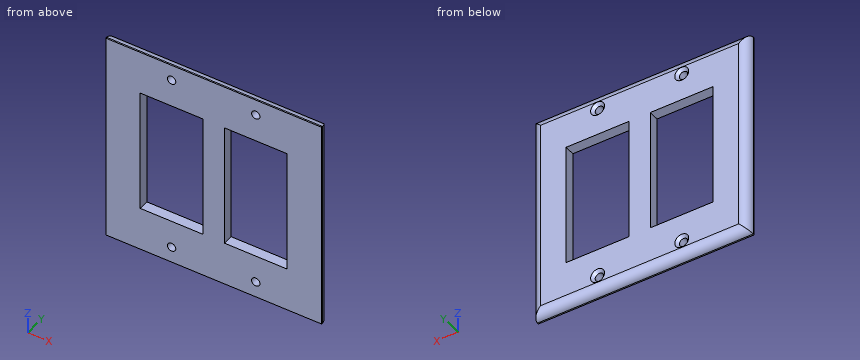
from build123d import *

# Parameters (mm, degrees)
SKETCH1_W           = 116
SKETCH1_H           = 114.3
SKETCH1_R           = 2.25
SKETCH1_W_2         = 33.75
SKETCH1_H_2         = 67
BOSS_EXTRUDE1_DEPTH = 5.5
FILLET1_R           = 4.75
CHAMFER1_SIZE       = 1.5


with BuildPart() as part:
    # Sketch1 → Boss-Extrude1 (new body)
    with BuildSketch(Plane(origin=(0, 0, 0), x_dir=(1, 0, 0), z_dir=(0, 1, 0))):
        with Locations((8.125405268, -27.177064496)):
            Rectangle(SKETCH1_W, SKETCH1_H)
        with Locations((-14.499594732, 21.322935504)):
            Circle(SKETCH1_R, mode=Mode.SUBTRACT)
        with Locations((-14.499594732, -75.677064496)):
            Circle(SKETCH1_R, mode=Mode.SUBTRACT)
        with Locations((30.750405268, -75.677064496)):
            Circle(SKETCH1_R, mode=Mode.SUBTRACT)
        with Locations((30.750405268, 21.322935504)):
            Circle(SKETCH1_R, mode=Mode.SUBTRACT)
        with Locations((-14.499594732, -27.177064496)):
            Rectangle(SKETCH1_W_2, SKETCH1_H_2, mode=Mode.SUBTRACT)
        with Locations((30.750405268, -27.177064496)):
            Rectangle(SKETCH1_W_2, SKETCH1_H_2, mode=Mode.SUBTRACT)
    extrude(amount=BOSS_EXTRUDE1_DEPTH)

    # Fillet1
    fillet1_edges = [part.edges().sort_by_distance(p)[0] for p in [
        (66.125405268, 5.5, 27.177064496),
        (8.125405268, 5.5, -29.972935504),
        (-49.874594732, 5.5, 27.177064496),
        (8.125405268, 5.5, 84.327064496),
    ]]
    fillet(fillet1_edges, radius=FILLET1_R)

    # Chamfer1
    chamfer1_edges = [part.edges().sort_by_distance(p)[0] for p in [
        (28.500405268, 5.5, 75.677064496),
        (-16.749594732, 5.5, 75.677064496),
        (-16.749594732, 5.5, -21.322935504),
        (28.500405268, 5.5, -21.322935504),
    ]]
    chamfer(chamfer1_edges, length=CHAMFER1_SIZE)


solid = part.part
CAD build for the part. Positions are in the model's coordinates, mm. Round coordinates to 2 decimals unless told otherwise and drop trailing zeros. Order: outer loops, then holes, each group sorted by start corner. A loop starts at its lowest first (then second) coordinate and runs counter-clockwise, first axis right, second up. Notation, with made-up numbers: (15, 19) -> (51, 19) arc R13 cw to (51, 30) -> close; hole circle Ø3 at (-21.5, 88). An arc over 180 degrees is marked (long way). Write item = value, one per line. Start each with the question number.
(1) Probe line 1 (X direction, y = 1.1, z = -2.5); line 2 (Z direction, x = -15.5, y = 3.5); line 3 (X direction, y = 0.5, z = 74). List the from-to ranges inside material, lowest first. Write a range as [from, to].
(2) Cut at C-C, the plane y = 2.15. List the corners of the cut face in (x, z), then the cut area to 3 significant figures.
(3) Cut at B-B, the plane x = -5. List the corners of the cut face in (y, z).
(4) Cut at D-D, the plane x = 10. List the corners of the cut face in (y, z).
(5) Pin check, flat tips, straight feed: P1, Ø3, axis at x = 25.5, y = 2.5, coming from the +Z side; P2, Ø5, axis at x = 30.75, z = 75.68, coming from the +Y side; P3, Ø2, axis at y = 2, z = -12.5, coming from the +X side; P4, Ø2.5, axis at x = -14.5, z = 75.68, coming from the -Y side. Stop position of each tip, or through.
(6) Cut at A-A, the plane z = 21. List the corners of the cut face in (x, y).
Model answer:
q1.line_1 = [-49.86, -31.37], [2.38, 13.88], [47.63, 66.11]
q1.line_2 = [-29.1, -23.34], [-19.31, -6.32], [60.68, 73.66], [77.69, 83.45]
q1.line_3 = [-49.87, -16], [-13, 29.25], [32.25, 66.13]
q2.outline = (-49.66, -29.76) -> (65.91, -29.76) -> (65.91, 84.12) -> (-49.66, 84.12) -> close; hole (-31.37, -6.32) -> (2.38, -6.32) -> (2.38, 60.68) -> (-31.37, 60.68) -> close; hole circle Ø4.5 at (-14.5, -21.32); hole circle Ø4.5 at (-14.5, 75.68); hole (13.88, -6.32) -> (47.63, -6.32) -> (47.63, 60.68) -> (13.88, 60.68) -> close; hole circle Ø4.5 at (30.75, -21.32); hole circle Ø4.5 at (30.75, 75.68)
q2.area = 8,580 mm2
q3.outline = (0, -29.97) -> (0.75, -29.97) arc R4.75 ccw to (5.5, -25.22) -> (5.5, -6.32) -> (0, -6.32) -> close; (0, 60.68) -> (5.5, 60.68) -> (5.5, 79.58) arc R4.75 ccw to (0.75, 84.33) -> (0, 84.33) -> close
q4.outline = (0, -29.97) -> (0.75, -29.97) arc R4.75 ccw to (5.5, -25.22) -> (5.5, 79.58) arc R4.75 ccw to (0.75, 84.33) -> (0, 84.33) -> close
q5.P1 = 84.32
q5.P2 = 4.25
q5.P3 = 66.12
q5.P4 = through
q6.outline = (-49.87, 0) -> (-31.37, 0) -> (-31.37, 5.5) -> (-45.12, 5.5) arc R4.75 ccw to (-49.87, 0.75) -> close; (2.38, 0) -> (13.88, 0) -> (13.88, 5.5) -> (2.38, 5.5) -> close; (47.63, 0) -> (66.13, 0) -> (66.13, 0.75) arc R4.75 ccw to (61.38, 5.5) -> (47.63, 5.5) -> close
